Could you check a few things on this model? Use its own coordinates, in mm. Face numbers are marked on the shaded views. A direction names the side the tool comes from. Coordinates: 2 decimals unless noted, no trailing zeros. Write each loop counter-clockwise with the first axis right and the second up, starting at its lowest first coordinate (ties: lowest second). Pieces come first, ordered by that corner, then holes. Notation, with made-up numbers: (-5.5, 67.5) - (28.5, 67.5) arc R25 ccw to (28.5, 104.5) - close; hole circle Ø7 at (12, 58.25). An arc over 180 degrees is marked (long way). Answer as a JSON object with one key per item and string values. Group by question number.
1) If we section it at B-B (x = 457): Write out the boundary of the cut face in (y, z), plus the area to 3 significant figures.
2) Please list where these lines run through material, in increasing order: line 1 along Z through (x, y) = (254.5, 293); line 2 along X through (y, z) = (294.5, 168); line 3 along Y through (x, z) = (317, 405.5).
3) If we section it at D-D (z = 83): Write out the boundary of the cut face in (x, y), plus the area to 3 significant figures.
4) Will these pins go through, and if not, where does the flat tip stop? pin 1 Ø8 at (y, z) = (639, 236) entering from +X; pin 2 Ø6 at (y, z) = (573, 305) entering from +X.
5) If we section it at A-A (z = 419.5): Write out the boundary of the cut face in (x, y), plus the area to 3 significant figures.
6) If we section it at C-C (y = 92.5): Write out the boundary of the cut face in (x, z), plus the area to 3 significant figures.
7) We'd pull the mould along X, two halves only. Please class the marked faces 1, 2 and 3: released by +X, released by -X, zero draft, split by the parting line, or undercut.
8) On a 3-axis mill with a long thin cutter (end or side, diameter ignored), from which of +Z, -Z, +X, -X, +Y, -Y can I reach the whole of each face in a straight line? I mean the marked faces 4, 5 and 6. Say none if no direction works.
```python
from build123d import *

# Parameters (mm, degrees)
BOSS_EXTRUDE1_DEPTH            = 508
SKETCH2_W                      = 175.72130466
SKETCH2_H                      = 449.160798253
CUT_EXTRUDE1_DEPTH             = 76.2
SKETCH3_W                      = 304.8
SKETCH3_H                      = 203.2
CUT_EXTRUDE3_DEPTH             = 50.8
SHELL2_START                   = 27.94
SHELL2_DEPTH                   = 452.12
SHELL2_2_DEPTH                 = 45.72
SHELL2_START_2                 = 434.34
SHELL2_3_DEPTH                 = 45.72
FILLET1_R                      = 7.62
CUT_EXTRUDE4_REACH             = 965.862
CUT_EXTRUDE4_DIRECTION_2_DEPTH = 97.536


# Read off the part's stored shape, not the designer's step: Shell2
with BuildPart() as part:
    # Sketch1 → Boss-Extrude1 (new body)
    with BuildSketch(Plane.XY):
        Polygon((508, 0), (508, 371.248348728), (279.4, 371.248348728), (83.128822626, 711.2), (0, 711.2), (0, 0), align=None)
    extrude(amount=BOSS_EXTRUDE1_DEPTH)

    # Sketch2 → Cut-Extrude1 (cut)
    with BuildSketch(Plane(origin=(0, 371.248348728, 0), x_dir=(1, 0, 0), z_dir=(0, 1, 0))):
        with Locations((387.505332687, -250.48614125)):
            Rectangle(SKETCH2_W, SKETCH2_H)
    extrude(amount=-CUT_EXTRUDE1_DEPTH, mode=Mode.SUBTRACT)

    # Sketch3 → Cut-Extrude3 (cut)
    with BuildSketch(Plane(origin=(370.305250556, 213.795836091, 0), x_dir=(0, 0, -1), z_dir=(0.8660254037844397, 0.49999999999999806, 0))):
        with Locations((-254, 371.152855858)):
            Rectangle(SKETCH3_W, SKETCH3_H)
    extrude(amount=-CUT_EXTRUDE3_DEPTH, mode=Mode.SUBTRACT)

    # Shell2 outline → Shell2 (cut)
    with BuildSketch(Plane.XY.offset(SHELL2_START)):
        Polygon((27.94, 27.94), (480.06, 27.94), (480.06, 267.108348728), (271.704680357, 267.108348728), (271.704680357, 343.308348728), (263.268833479, 343.308348728), (225.302072845, 409.068707145), (205.504732114, 397.638707145), (191.534732114, 421.835456927), (89.934732114, 597.811818976), (75.964732114, 622.008568757), (95.762072845, 633.438568757), (66.997656105, 683.26), (27.94, 683.26), align=None)
    extrude(amount=SHELL2_DEPTH, mode=Mode.SUBTRACT)

    # Shell2 2 outline → Shell2 2 (cut)
    with BuildSketch(Plane.XY.offset(SHELL2_START)):
        Polygon((225.302072845, 409.068707145), (95.762072845, 633.438568757), (75.964732114, 622.008568757), (89.934732114, 597.811818976), (191.534732114, 421.835456927), (205.504732114, 397.638707145), align=None)
    extrude(amount=SHELL2_2_DEPTH, mode=Mode.SUBTRACT)

    # Shell2 3 outline → Shell2 3 (cut)
    with BuildSketch(Plane.XY.offset(SHELL2_START_2)):
        Polygon((225.302072845, 409.068707145), (95.762072845, 633.438568757), (75.964732114, 622.008568757), (89.934732114, 597.811818976), (191.534732114, 421.835456927), (205.504732114, 397.638707145), align=None)
    extrude(amount=SHELL2_3_DEPTH, mode=Mode.SUBTRACT)

    # Fillet1
    fillet1_edges = [part.edges().sort_by_distance(p)[0] for p in [
        (393.7, 371.248348728, 508),
        (181.264411313, 541.224174364, 508),
        (41.564411313, 711.2, 508),
        (508, 185.624174364, 508),
    ]]
    fillet(fillet1_edges, radius=FILLET1_R)

    # Cut-Extrude4: up to this face of the body (flat: up to its plane)
    cut_extrude4_end = Plane(part.part.faces().sort_by_distance((162.73177737, 522.523637951, 101.6))[0])
    # Sketch6 → Cut-Extrude4 (cut, up to the picked face)
    with BuildSketch(Plane(origin=(0, 0, 406.4), x_dir=(-1, 0, 0), z_dir=(0, 0, -1)), mode=Mode.PRIVATE) as cut_extrude4_sk1:
        Polygon((-109.711824261, 652.442307464), (-240.02087993, 424.214985446), (-218.44952186, 411.898566558), (-97.827125151, 645.656599669), align=None)
    cut_extrude4_tool1 = split(extrude(cut_extrude4_sk1.sketch, amount=CUT_EXTRUDE4_REACH, mode=Mode.PRIVATE), bisect_by=cut_extrude4_end, keep=Keep.BOTH, mode=Mode.PRIVATE)
    add(cut_extrude4_tool1.solids().sort_by(Axis((172.556766, 522.406417, 406.4), (0, 0, -1)))[0], mode=Mode.SUBTRACT)

    # Sketch6 → Cut-Extrude4 direction 2 (cut)
    with BuildSketch(Plane(origin=(0, 0, 406.4), x_dir=(-1, 0, 0), z_dir=(0, 0, -1))):
        Polygon((-109.711824261, 652.442307464), (-240.02087993, 424.214985446), (-218.44952186, 411.898566558), (-97.827125151, 645.656599669), align=None)
    extrude(amount=-CUT_EXTRUDE4_DIRECTION_2_DEPTH, mode=Mode.SUBTRACT)


solid = part.part
```
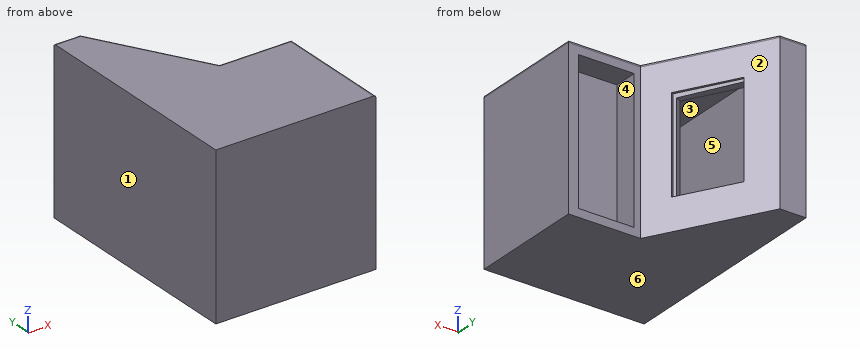
Here are the results:
{
 "1": {"outline": "(0, 0) - (371.25, 0) - (371.25, 25.91) - (295.05, 25.91) - (295.05, 475.07) - (371.25, 475.07) - (371.25, 500.38) arc R7.62 ccw to (363.63, 508) - (0, 508) - close; hole (27.94, 27.94) - (267.11, 27.94) - (267.11, 480.06) - (27.94, 480.06) - close", "area": "46,200 mm²"},
 "2": {"line 1": "z = 0 to 27.94, 480.06 to 508", "line 2": "x = 0 to 27.94, 271.7 to 508", "line 3": "y = 0 to 27.94, 267.11 to 295.05"},
 "3": {"outline": "(0, 0) - (508, 0) - (508, 371.25) - (475.37, 371.25) - (475.37, 295.05) - (299.64, 295.05) - (299.64, 371.25) - (279.4, 371.25) - (83.13, 711.2) - (0, 711.2) - close; hole (27.94, 27.94) - (480.06, 27.94) - (480.06, 267.11) - (271.7, 267.11) - (271.7, 343.31) - (263.27, 343.31) - (225.3, 409.07) - (205.5, 397.64) - (75.96, 622.01) - (95.76, 633.44) - (67, 683.26) - (27.94, 683.26) - close", "area": "69,400 mm²"},
 "4": {"pin 1": "stops at x = 127.12", "pin 2": "stops at x = 27.94"},
 "5": {"outline": "(0, 0) - (508, 0) - (508, 371.25) - (475.37, 371.25) - (475.37, 295.05) - (299.64, 295.05) - (299.64, 371.25) - (279.4, 371.25) - (83.13, 711.2) - (0, 711.2) - close; hole (27.94, 27.94) - (480.06, 27.94) - (480.06, 267.11) - (271.7, 267.11) - (271.7, 343.31) - (263.27, 343.31) - (225.3, 409.07) - (205.5, 397.64) - (75.96, 622.01) - (95.76, 633.44) - (67, 683.26) - (27.94, 683.26) - close; hole (97.83, 645.66) - (218.45, 411.9) - (240.02, 424.21) - (109.71, 652.44) - close", "area": "64,300 mm²"},
 "6": {"outline": "(0, 0) - (508, 0) - (508, 500.38) arc R7.62 ccw to (500.38, 508) - (0, 508) - close; hole (27.94, 27.94) - (480.06, 27.94) - (480.06, 480.06) - (27.94, 480.06) - close", "area": "53,600 mm²"},
 "7": {"face 1": "released by -X", "face 2": "released by +X", "face 3": "undercut"},
 "8": {"face 4": "+Y", "face 5": "none", "face 6": "-Z, +X, -X, +Y, -Y"}
}
